from build123d import *

# Parameters (mm, degrees)
SKETCH1_W           = 49
SKETCH1_H           = 28
BOSS_EXTRUDE1_DEPTH = 45
SKETCH2_W           = 43
SKETCH2_H           = 22
CUT_EXTRUDE1_DEPTH  = 43
SKETCH3_W           = 29
SKETCH3_H           = 8
CUT_EXTRUDE2_DEPTH  = 3
SKETCH4_R           = 1.5
CUT_EXTRUDE3_DEPTH  = 3
BOSS_EXTRUDE2_DEPTH = 45
SKETCH6_R           = 1.49
CUT_EXTRUDE4_DEPTH  = 45
BOSS_EXTRUDE3_DEPTH = 45
SKETCH8_R           = 1.49
CUT_EXTRUDE5_DEPTH  = 45
FILLET2_R           = 1


with BuildPart() as part:
    # Sketch1 → Boss-Extrude1 (new body)
    with BuildSketch(Plane(origin=(0, 0, 0), x_dir=(1, 0, 0), z_dir=(0, 1, 0))):
        with Locations((-4.986725664, 3.221238938)):
            Rectangle(SKETCH1_W, SKETCH1_H)
    extrude(amount=BOSS_EXTRUDE1_DEPTH)

    # Sketch2 → Cut-Extrude1 (cut)
    with BuildSketch(Plane(origin=(0, 45, 0), x_dir=(1, 0, 0), z_dir=(0, 1, 0))):
        with Locations((-4.986725664, 3.221238938)):
            Rectangle(SKETCH2_W, SKETCH2_H)
    extrude(amount=-CUT_EXTRUDE1_DEPTH, mode=Mode.SUBTRACT)

    # Sketch3 → Cut-Extrude2 (cut)
    with BuildSketch(Plane(origin=(0, 2, 0), x_dir=(1, 0, 0), z_dir=(0, 1, 0))):
        with Locations((-4.986725664, 7.221238938)):
            Rectangle(SKETCH3_W, SKETCH3_H)
    extrude(amount=-CUT_EXTRUDE2_DEPTH, mode=Mode.SUBTRACT)

    # Sketch4 → Cut-Extrude3 (cut)
    with BuildSketch(Plane.XY.offset(-14.221238938)):
        with Locations((-2.986725664, 35)):
            Circle(SKETCH4_R)
    extrude(amount=-CUT_EXTRUDE3_DEPTH, mode=Mode.SUBTRACT)

    # Sketch5 → Boss-Extrude2 (add)
    with BuildSketch(Plane.XZ):
        with BuildLine():
            Line((14.867523025, 10.778761062), (19.513274336, 10.778761062))
            Line((19.513274336, 10.778761062), (19.513274336, 6.133009751))
            ThreePointArc((19.513274336, 6.133009751), (14.093718863, 5.359205589), (14.867523025, 10.778761062))
        make_face()
    extrude(amount=-BOSS_EXTRUDE2_DEPTH)

    # Sketch6 → Cut-Extrude4 (cut)
    with BuildSketch(Plane.XZ):
        with Locations((16.513274336, 7.778761062)):
            Circle(SKETCH6_R)
    extrude(amount=-CUT_EXTRUDE4_DEPTH, mode=Mode.SUBTRACT)

    # Sketch7 → Boss-Extrude3 (add)
    with BuildSketch(Plane.XZ):
        with BuildLine():
            Line((-29.486725664, 5.133009751), (-29.486725664, 10.778761062))
            Line((-29.486725664, 10.778761062), (-23.840974353, 10.778761062))
            ThreePointArc((-23.840974353, 10.778761062), (-23.658298539, 4.950333937), (-29.486725664, 5.133009751))
        make_face()
    extrude(amount=-BOSS_EXTRUDE3_DEPTH)

    # Sketch8 → Cut-Extrude5 (cut)
    with BuildSketch(Plane.XZ):
        with Locations((-26.486725664, 7.778761062)):
            Circle(SKETCH8_R)
    extrude(amount=-CUT_EXTRUDE5_DEPTH, mode=Mode.SUBTRACT)

    # Fillet2
    fillet2_edges = [part.edges().sort_by_distance(p)[0] for p in [
        (-4.986725664, 0, -17.221238938),
        (19.513274336, 0, -3.221238938),
        (-4.986725664, 0, 10.778761062),
        (-29.486725664, 0, -3.221238938),
        (-29.486725664, 22.5, -17.221238938),
        (19.513274336, 22.5, -17.221238938),
        (19.513274336, 22.5, 10.778761062),
        (-29.486725664, 22.5, 10.778761062),
    ]]
    fillet(fillet2_edges, radius=FILLET2_R)


solid = part.part
The listing builds one solid part. Answer for the finished solid, in the listing's coordinates (mm). A direction names the side the tool comes from. Coordinates: 2 decimals unless noted, no trailing zeros. Order: outer loops, then holes, each group sorted by start corner. A loop starts at its lowest first (then second) coordinate and runs counter-clockwise, first axis right, second up. Notation, with made-up numbers: (10.5, 23.5) -> (22.5, 23.5) arc R14 ccw to (22.5, 33.5) -> close; hole circle Ø5 at (80.5, -18). An arc over 180 degrees is marked (long way). Answer in a Markdown table with one row per item. Add a question column.
Item 1: Find the intervals of material crossed by L1, parallel to Z at x = -9, y = 8; L2, parallel to X at y = 42.5, z = -0.75; L3, parallel to Z at x = 15.5, y = 29.5, in increasing order. Write a range as from..to.
Item 2: Find section D-D (y = 35). Write down the section's boundary in (x, z), then the cut area to 3 significant figures.
Item 3: Which of the six approach directions +Z, -Z, +X, -X, +Y, -Y give full straight-line access (tool end or side, diameter ignored) to faces 1 (the face through (-3.312, 33.536, -15.7)), 2 (the face through (-26.487, 24, -5)), 3 (the face through (-5, 1, -11.221)), 4 (the face through (-5, 23, -17.221)), 5 (the face through (-5, 0, -1))?
Item 4: Each of these flat-tipped pins is pushed along its axis until it touches: P1, Ø1.5, axis at x = -3.5, z = -2.5, coming from the +Y side; P2, Ø1.8, axis at x = -2.99, y = 35, coming from the -Z side. Where does it stop, or does it pass through?
Item 5: Find section A-A (x = 8). Write down the section's boundary in (y, z).
Item 6: Determine the mould class of faces 6 (the face through (-3, 45, 8)), 7 (the face through (-5, 23, 10.779)), 8 (the face through (-27.975, 22.185, 7.844)) for opening direction Z: +Z half, -Z half, draft (parallel to the pull), parting line (faces both ways), or undercut.
Item 7: Find section C-C (z = 2.25). Write down the section's boundary in (x, y).
Item 8: Find section B-B (y = 6). Write down the section's boundary in (x, z), then the cut area to 3 significant figures.
Result set:
| question | item | result |
|---|---|---|
| 1 | L1 | z = -17.22..-14.22, 7.78..10.78 |
| 1 | L2 | x = -29.49..-26.49, 16.51..19.51 |
| 1 | L3 | z = -17.22..-14.22, 4.51..6.69, 8.87..10.78 |
| 2 | outline | (-29.49, -16.22) arc R1 ccw to (-28.49, -17.22) -> (-4.49, -17.22) -> (-4.49, -14.22) -> (-26.49, -14.22) -> (-26.49, 3.78) arc R4 ccw to (-22.49, 7.78) -> (13.09, 7.78) arc R3.42 ccw to (16.51, 4.36) -> (16.51, -14.22) -> (-1.49, -14.22) -> (-1.49, -17.22) -> (18.51, -17.22) arc R1 ccw to (19.51, -16.22) -> (19.51, 9.78) arc R1 ccw to (18.51, 10.78) -> (-28.49, 10.78) arc R1 ccw to (-29.49, 9.78) -> close; hole circle Ø2.98 at (-26.49, 7.78); hole circle Ø2.98 at (16.51, 7.78) |
| 2 | area | 424 mm² |
| 3 | face 1 | -Z |
| 3 | face 2 | +Y |
| 3 | face 3 | +Y, -Y |
| 3 | face 4 | -Z, +X, -X, +Y, -Y |
| 3 | face 5 | +Z, -Z, +X, -X, -Y |
| 4 | P1 | stops at y = 2 |
| 4 | P2 | stops at z = 7.78 |
| 5 | outline | (0, -16.22) arc R1 ccw to (1, -17.22) -> (45, -17.22) -> (45, -14.22) -> (2, -14.22) -> (2, -11.22) -> (0, -11.22) -> close; (0, -3.22) -> (2, -3.22) -> (2, 7.78) -> (45, 7.78) -> (45, 10.78) -> (1, 10.78) arc R1 ccw to (0, 9.78) -> close |
| 6 | face 6 | draft |
| 6 | face 7 | +Z half |
| 6 | face 8 | undercut |
| 7 | outline | (-29.49, 1) arc R1 ccw to (-28.49, 0) -> (18.51, 0) arc R1 ccw to (19.51, 1) -> (19.51, 45) -> (16.51, 45) -> (16.51, 2) -> (-26.49, 2) -> (-26.49, 45) -> (-29.49, 45) -> close |
| 8 | outline | (-29.49, -16.22) arc R1 ccw to (-28.49, -17.22) -> (18.51, -17.22) arc R1 ccw to (19.51, -16.22) -> (19.51, 9.78) arc R1 ccw to (18.51, 10.78) -> (-28.49, 10.78) arc R1 ccw to (-29.49, 9.78) -> close; hole circle Ø2.98 at (-26.49, 7.78); hole (-26.49, -14.22) -> (16.51, -14.22) -> (16.51, 4.36) arc R3.42 cw to (13.09, 7.78) -> (-22.49, 7.78) arc R4 cw to (-26.49, 3.78) -> close; hole circle Ø2.98 at (16.51, 7.78) |
| 8 | area | 433 mm² |
